```python
from build123d import *

# Parameters (mm, degrees)
BOSS_EXTRUDE1_DEPTH = 10
SKETCH2_R           = 2.5
BOSS_EXTRUDE2_DEPTH = 5
SKETCH3_R           = 2.5
BOSS_EXTRUDE3_DEPTH = 25
SKETCH5_R           = 2.5
CUT_EXTRUDE1_DEPTH  = 5
SKETCH4_R           = 2.5
CUT_EXTRUDE2_DEPTH  = 5


with BuildPart() as part:
    # Sketch1 → Boss-Extrude1 (new body)
    with BuildSketch(Plane(origin=(0, 0, 0), x_dir=(1, 0, 0), z_dir=(0, 1, 0))):
        with BuildLine():
            Line((-22.5, -5), (22.5, -5))
            ThreePointArc((22.5, -5), (27.5, 0), (22.5, 5))
            Line((22.5, 5), (-22.5, 5))
            ThreePointArc((-22.5, 5), (-27.5, 0), (-22.5, -5))
        make_face()
    extrude(amount=BOSS_EXTRUDE1_DEPTH)

    # Sketch2 → Boss-Extrude2 (add)
    with BuildSketch(Plane(origin=(0, 10, 0), x_dir=(1, 0, 0), z_dir=(0, 1, 0))):
        with Locations((-22.5, 0)):
            Circle(SKETCH2_R)
    extrude(amount=BOSS_EXTRUDE2_DEPTH)

    # Sketch3 → Boss-Extrude3 (add)
    with BuildSketch(Plane(origin=(0, 10, 0), x_dir=(1, 0, 0), z_dir=(0, 1, 0))):
        with Locations((22.5, 0)):
            Circle(SKETCH3_R)
    extrude(amount=-BOSS_EXTRUDE3_DEPTH)

    # Sketch5 → Cut-Extrude1 (cut)
    with BuildSketch(Plane.XZ):
        with Locations((-22.5, 0)):
            Circle(SKETCH5_R)
    extrude(amount=-CUT_EXTRUDE1_DEPTH, mode=Mode.SUBTRACT)

    # Sketch4 → Cut-Extrude2 (cut)
    with BuildSketch(Plane(origin=(0, 10, 0), x_dir=(1, 0, 0), z_dir=(0, 1, 0))):
        with Locations((22.5, 0)):
            Circle(SKETCH4_R)
    extrude(amount=-CUT_EXTRUDE2_DEPTH, mode=Mode.SUBTRACT)


solid = part.part
```
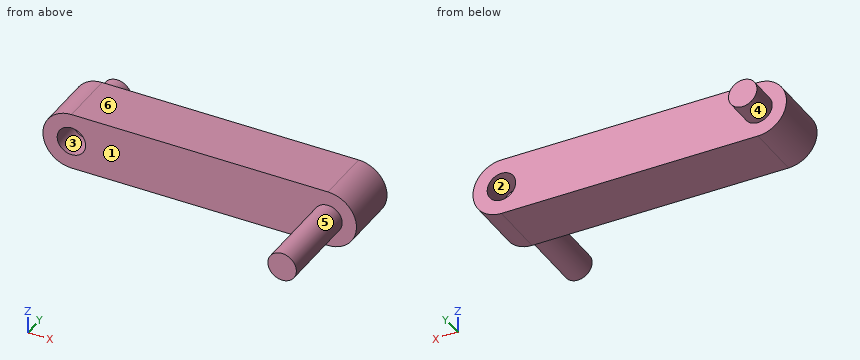
Work out the finished part from the listing and answer in its coordinate system (mm). Face numbers are marked on the shaded views. A direction names the side the tool comes from. Coordinates: 2 decimals unless noted, no trailing zeros. Loops run counter-clockwise (first coordinate to the right, second up) from the corner with the lowest first, then second, coordinate; pieces in that order, holes last.
1) Section C-C (x = 17.5) is taken. Give the vertices of the cut face in (y, z).
Results:
outline: (0, -5) - (10, -5) - (10, 5) - (0, 5) - close
2) For a pull along X with two mould halves and no side action, classify the marked faces 1, 2, 3 and 4 as +X half, -X half, draft (parallel to the pull), parting line (faces both ways), or undercut.
Results:
face 1: draft
face 2: undercut
face 3: undercut
face 4: parting line
3) Section A-A (y = 9) is taken. Give the vertices of the cut face in (x, z), plus the area to 3 significant figures.
Results:
outline: (-22.5, -5) - (22.5, -5) arc R5 ccw to (22.5, 5) - (-22.5, 5) arc R5 ccw to start; hole circle Ø5 at (22.5, 0)
area: 509 mm2
4) Section D-D (z = -3.25) is taken. Give the vertices of the cut face in (x, y), plus the area to 3 significant figures.
Results:
outline: (-26.3, 0) - (26.3, 0) - (26.3, 10) - (-26.3, 10) - close
area: 526 mm2
5) Section B-B (z = 0) is taken. Give the vertices of the cut face in (x, y).
Results:
outline: (-27.5, 0) - (-25, 0) - (-25, 5) - (-20, 5) - (-20, 0) - (20, 0) - (20, -15) - (25, -15) - (25, 0) - (27.5, 0) - (27.5, 10) - (25, 10) - (25, 5) - (20, 5) - (20, 10) - (-20, 10) - (-20, 15) - (-25, 15) - (-25, 10) - (-27.5, 10) - close
6) Consider probe 1 along Z at (x, y) = (22.5, 8.05); probe 2 along Y at (x, z) = (7.5, -1.5); probe 3 along Y at (x, z) = (23, 0). Determine where each line is inside the solid, lowest interval first.
Results:
probe 1: z = -5 to -2.5, 2.5 to 5
probe 2: y = 0 to 10
probe 3: y = -15 to 5
7) For the marked faces 5 and 6, determine the directions among +Z, -Z, +X, -X, +Y, -Y from which every point of the face is accessible in a straight line to the end or side of a thin tool.
Results:
face 5: -Y
face 6: +Z, +X, -X, +Y, -Y
8) Flat-ended cylindrical pins translate along their axes: pin 1 (4 mm diameter, centred on x = 23.5, z = -0.5, fed in from +Y); pin 2 (1.5 mm diameter, centred on y = 10.5, z = -1, fed in from +X); pin 3 (4 mm diameter, centred on y = -5, z = -2, fed in from +X). Find the tip coordinate at first contact, or state that the pin passes through.
Results:
pin 1: stops at y = 10
pin 2: stops at x = 27.48
pin 3: stops at x = 25
